from build123d import *

# Parameters (mm, degrees)
CONVERT_SOLID1_START = -1.5
CONVERT_SOLID1_DEPTH = 1.5


# Read off the part's stored shape, not the designer's step: Convert-Solid1
with BuildPart() as part:
    # Convert-Solid1 outline → Convert-Solid1 (new body)
    with BuildSketch(Plane.XY.offset(CONVERT_SOLID1_START)):
        with BuildLine():
            ThreePointArc((374, 0), (375.414213562, 0.585786438), (376, 2))
            Line((376, 2), (376, 480))
            ThreePointArc((376, 480), (375.414213562, 481.414213562), (374, 482))
            Line((374, 482), (2, 482))
            ThreePointArc((2, 482), (0.585786438, 481.414213562), (0, 480))
            Line((0, 480), (0, 2))
            ThreePointArc((0, 2), (0.585786438, 0.585786438), (2, 0))
            Line((2, 0), (50.458688877, 0))
            ThreePointArc((50.458688877, 0), (51.382309639, 0.226042647), (52.097152718, 0.853075311))
            Line((52.097152718, 0.853075311), (82.402847282, 44.146924689))
            ThreePointArc((82.402847282, 44.146924689), (83.117690361, 44.773957353), (84.041311123, 45))
            Line((84.041311123, 45), (291.958688877, 45))
            ThreePointArc((291.958688877, 45), (292.882309639, 44.773957353), (293.597152718, 44.146924689))
            Line((293.597152718, 44.146924689), (323.902847282, 0.853075311))
            ThreePointArc((323.902847282, 0.853075311), (324.617690361, 0.226042647), (325.541311123, 0))
            Line((325.541311123, 0), (374, 0))
        make_face()
        with BuildLine():
            Line((23, 23.65), (24, 23.65))
            ThreePointArc((24, 23.65), (25.65, 22), (24, 20.35))
            Line((24, 20.35), (23, 20.35))
            ThreePointArc((23, 20.35), (21.35, 22), (23, 23.65))
        make_face(mode=Mode.SUBTRACT)
        with BuildLine():
            Line((23, 98.65), (24, 98.65))
            ThreePointArc((24, 98.65), (25.65, 97), (24, 95.35))
            Line((24, 95.35), (23, 95.35))
            ThreePointArc((23, 95.35), (21.35, 97), (23, 98.65))
        make_face(mode=Mode.SUBTRACT)
        with BuildLine():
            Line((23, 173.65), (24, 173.65))
            ThreePointArc((24, 173.65), (25.65, 172), (24, 170.35))
            Line((24, 170.35), (23, 170.35))
            ThreePointArc((23, 170.35), (21.35, 172), (23, 173.65))
        make_face(mode=Mode.SUBTRACT)
        with BuildLine():
            Line((352, 23.65), (353, 23.65))
            ThreePointArc((353, 23.65), (354.65, 22), (353, 20.35))
            Line((353, 20.35), (352, 20.35))
            ThreePointArc((352, 20.35), (350.35, 22), (352, 23.65))
        make_face(mode=Mode.SUBTRACT)
        with BuildLine():
            Line((352, 98.65), (353, 98.65))
            ThreePointArc((353, 98.65), (354.65, 97), (353, 95.35))
            Line((353, 95.35), (352, 95.35))
            ThreePointArc((352, 95.35), (350.35, 97), (352, 98.65))
        make_face(mode=Mode.SUBTRACT)
        with BuildLine():
            Line((302.5, 75), (73.5, 75))
            ThreePointArc((73.5, 75), (66.428932188, 77.928932188), (63.5, 85))
            Line((63.5, 85), (63.5, 292))
            ThreePointArc((63.5, 292), (66.428932188, 299.071067812), (73.5, 302))
            Line((73.5, 302), (302.5, 302))
            ThreePointArc((302.5, 302), (309.571067812, 299.071067812), (312.5, 292))
            Line((312.5, 292), (312.5, 85))
            ThreePointArc((312.5, 85), (309.571067812, 77.928932188), (302.5, 75))
        make_face(mode=Mode.SUBTRACT)
        with BuildLine():
            Line((352, 173.65), (353, 173.65))
            ThreePointArc((353, 173.65), (354.65, 172), (353, 170.35))
            Line((353, 170.35), (352, 170.35))
            ThreePointArc((352, 170.35), (350.35, 172), (352, 173.65))
        make_face(mode=Mode.SUBTRACT)
        with BuildLine():
            Line((23, 248.65), (24, 248.65))
            ThreePointArc((24, 248.65), (25.65, 247), (24, 245.35))
            Line((24, 245.35), (23, 245.35))
            ThreePointArc((23, 245.35), (21.35, 247), (23, 248.65))
        make_face(mode=Mode.SUBTRACT)
        with BuildLine():
            Line((23, 323.65), (24, 323.65))
            ThreePointArc((24, 323.65), (25.65, 322), (24, 320.35))
            Line((24, 320.35), (23, 320.35))
            ThreePointArc((23, 320.35), (21.35, 322), (23, 323.65))
        make_face(mode=Mode.SUBTRACT)
        with BuildLine():
            Line((7.98683607, 345.178083895), (8.98683607, 345.178083895))
            ThreePointArc((8.98683607, 345.178083895), (11.08683607, 343.078083895), (8.98683607, 340.978083895))
            Line((8.98683607, 340.978083895), (7.98683607, 340.978083895))
            ThreePointArc((7.98683607, 340.978083895), (5.88683607, 343.078083895), (7.98683607, 345.178083895))
        make_face(mode=Mode.SUBTRACT)
        with BuildLine():
            Line((21.48683607, 345.178083895), (22.48683607, 345.178083895))
            ThreePointArc((22.48683607, 345.178083895), (24.58683607, 343.078083895), (22.48683607, 340.978083895))
            Line((22.48683607, 340.978083895), (21.48683607, 340.978083895))
            ThreePointArc((21.48683607, 340.978083895), (19.38683607, 343.078083895), (21.48683607, 345.178083895))
        make_face(mode=Mode.SUBTRACT)
        with BuildLine():
            Line((6.48683607, 372.678083895), (7.48683607, 372.678083895))
            ThreePointArc((7.48683607, 372.678083895), (9.58683607, 370.578083895), (7.48683607, 368.478083895))
            Line((7.48683607, 368.478083895), (6.48683607, 368.478083895))
            ThreePointArc((6.48683607, 368.478083895), (4.38683607, 370.578083895), (6.48683607, 372.678083895))
        make_face(mode=Mode.SUBTRACT)
        with BuildLine():
            Line((36.48683607, 367.728083895), (37.48683607, 367.728083895))
            ThreePointArc((37.48683607, 367.728083895), (39.13683607, 366.078083895), (37.48683607, 364.428083895))
            Line((37.48683607, 364.428083895), (36.48683607, 364.428083895))
            ThreePointArc((36.48683607, 364.428083895), (34.83683607, 366.078083895), (36.48683607, 367.728083895))
        make_face(mode=Mode.SUBTRACT)
        with BuildLine():
            Line((23, 398.65), (24, 398.65))
            ThreePointArc((24, 398.65), (25.65, 397), (24, 395.35))
            Line((24, 395.35), (23, 395.35))
            ThreePointArc((23, 395.35), (21.35, 397), (23, 398.65))
        make_face(mode=Mode.SUBTRACT)
        with BuildLine():
            Line((23, 473.65), (24, 473.65))
            ThreePointArc((24, 473.65), (25.65, 472), (24, 470.35))
            Line((24, 470.35), (23, 470.35))
            ThreePointArc((23, 470.35), (21.35, 472), (23, 473.65))
        make_face(mode=Mode.SUBTRACT)
        with BuildLine():
            Line((105.25, 473.65), (106.25, 473.65))
            ThreePointArc((106.25, 473.65), (107.9, 472), (106.25, 470.35))
            Line((106.25, 470.35), (105.25, 470.35))
            ThreePointArc((105.25, 470.35), (103.6, 472), (105.25, 473.65))
        make_face(mode=Mode.SUBTRACT)
        with BuildLine():
            Line((352, 248.65), (353, 248.65))
            ThreePointArc((353, 248.65), (354.65, 247), (353, 245.35))
            Line((353, 245.35), (352, 245.35))
            ThreePointArc((352, 245.35), (350.35, 247), (352, 248.65))
        make_face(mode=Mode.SUBTRACT)
        with BuildLine():
            Line((352, 323.65), (353, 323.65))
            ThreePointArc((353, 323.65), (354.65, 322), (353, 320.35))
            Line((353, 320.35), (352, 320.35))
            ThreePointArc((352, 320.35), (350.35, 322), (352, 323.65))
        make_face(mode=Mode.SUBTRACT)
        with BuildLine():
            Line((355.01316393, 345.178083895), (356.01316393, 345.178083895))
            ThreePointArc((356.01316393, 345.178083895), (358.11316393, 343.078083895), (356.01316393, 340.978083895))
            Line((356.01316393, 340.978083895), (355.01316393, 340.978083895))
            ThreePointArc((355.01316393, 340.978083895), (352.91316393, 343.078083895), (355.01316393, 345.178083895))
        make_face(mode=Mode.SUBTRACT)
        with BuildLine():
            Line((367.01316393, 345.178083895), (368.01316393, 345.178083895))
            ThreePointArc((368.01316393, 345.178083895), (370.11316393, 343.078083895), (368.01316393, 340.978083895))
            Line((368.01316393, 340.978083895), (367.01316393, 340.978083895))
            ThreePointArc((367.01316393, 340.978083895), (364.91316393, 343.078083895), (367.01316393, 345.178083895))
        make_face(mode=Mode.SUBTRACT)
        with BuildLine():
            Line((187.5, 473.65), (188.5, 473.65))
            ThreePointArc((188.5, 473.65), (190.15, 472), (188.5, 470.35))
            Line((188.5, 470.35), (187.5, 470.35))
            ThreePointArc((187.5, 470.35), (185.85, 472), (187.5, 473.65))
        make_face(mode=Mode.SUBTRACT)
        with BuildLine():
            Line((269.75, 473.65), (270.75, 473.65))
            ThreePointArc((270.75, 473.65), (272.4, 472), (270.75, 470.35))
            Line((270.75, 470.35), (269.75, 470.35))
            ThreePointArc((269.75, 470.35), (268.1, 472), (269.75, 473.65))
        make_face(mode=Mode.SUBTRACT)
        with BuildLine():
            Line((361.51316393, 367.728083895), (362.51316393, 367.728083895))
            ThreePointArc((362.51316393, 367.728083895), (364.16316393, 366.078083895), (362.51316393, 364.428083895))
            Line((362.51316393, 364.428083895), (361.51316393, 364.428083895))
            ThreePointArc((361.51316393, 364.428083895), (359.86316393, 366.078083895), (361.51316393, 367.728083895))
        make_face(mode=Mode.SUBTRACT)
        with BuildLine():
            Line((368.51316393, 372.678083895), (369.51316393, 372.678083895))
            ThreePointArc((369.51316393, 372.678083895), (371.61316393, 370.578083895), (369.51316393, 368.478083895))
            Line((369.51316393, 368.478083895), (368.51316393, 368.478083895))
            ThreePointArc((368.51316393, 368.478083895), (366.41316393, 370.578083895), (368.51316393, 372.678083895))
        make_face(mode=Mode.SUBTRACT)
        with BuildLine():
            Line((352, 398.65), (353, 398.65))
            ThreePointArc((353, 398.65), (354.65, 397), (353, 395.35))
            Line((353, 395.35), (352, 395.35))
            ThreePointArc((352, 395.35), (350.35, 397), (352, 398.65))
        make_face(mode=Mode.SUBTRACT)
        with BuildLine():
            Line((352, 473.65), (353, 473.65))
            ThreePointArc((353, 473.65), (354.65, 472), (353, 470.35))
            Line((353, 470.35), (352, 470.35))
            ThreePointArc((352, 470.35), (350.35, 472), (352, 473.65))
        make_face(mode=Mode.SUBTRACT)
    extrude(amount=CONVERT_SOLID1_DEPTH)


solid = part.part
For this review, take the finished solid that the model builds, in its own axes (mm). A direction names the side the tool comes from. Give positions to 0.01 mm unless a question says otherwise; leave off trailing zeros. Loops run counter-clockwise (first coordinate to the right, second up) from the corner with the lowest first, then second, coordinate; pieces in that order, holes last. Notation, with made-up numbers: M -14,50.5 L 29,50.5 A5 cw 29,54.5 Z; hole C 72.5,18.5 d9. An arc over 180 degrees is marked long. Put each result on its own line as item: value. Start each with the question number.
(1) The part is to be moulded in two halves that separate along Y. For faces 1 (the cylindrical face through (309.65, 78.01, -0.76)), 2 (the flat face through (185, 351, 0)), 3 (the flat face through (67.04, 22.2, -0.76)), say which applies: +Y half, -Y half, draft (parallel to the pull), parting line (faces both ways), or undercut.
(2) Add section A-A, the plane x = 245.5. Write out the cut boundary in (y, z), then the cut area to 3 significant figures.
(3) For pin 1 (0.5 mm diameter, centred on x = 188, z = -0.5, fed in from -Y), flat-tipped, find the tip position at first contact; note if it passes through.
(4) Add section B-B, the plane y = 265.5. Write out the cut boundary in (x, z).
(5) Add section C-C, the plane z = -0.9. Give the number of separate pieces and of enclosed holes in the cut face, then the cut area to 3 significant figures.
(6) Machinability: for faces 4 (the cylindrical face through (66.35, 298.99, -0.76)), 5 (the flat face through (185, 351, -1.5)), 6 (the flat face through (308.54, 22.8, -0.76)), which of the approach directions +Z, -Z, +X, -X, +Y, -Y give a long, thin tool a straight path to every point of the face, cutting with its end or side? Answer none if there is none.
(7) Wall thickness on L1, parallel to X at y = 175.5, z = -0.85; L2, parallel to Y at x = 183.5, z = -1.1: over which ranges is each line inside the solid? List them lowest first.
Result:
1. face 1: undercut
1. face 2: draft
1. face 3: -Y half
2. outline: M 45,-1.5 L 75,-1.5 L 75,0 L 45,0 Z; M 302,-1.5 L 482,-1.5 L 482,0 L 302,0 Z
2. area: 315 mm^2
3. pin 1: stops at y = 45
4. outline: M 0,-1.5 L 63.5,-1.5 L 63.5,0 L 0,0 Z; M 312.5,-1.5 L 376,-1.5 L 376,0 L 312.5,0 Z
5. separate pieces: 1
5. enclosed holes: 26
5. area: 114,000 mm^2
6. face 4: +Z, -Z
6. face 5: -Z, +X, -X, +Y, -Y
6. face 6: +Z, -Z, -Y
7. L1: x = 0 to 63.5, 312.5 to 376
7. L2: y = 45 to 75, 302 to 482
